CAD build for the part. Positions are in the model's coordinates, mm. Give positions to 0.01 mm unless a question says otherwise; leave off trailing zeros. Loops run counter-clockwise (first coordinate to the right, second up) from the corner with the lowest first, then second, coordinate; pieces in that order, holes last. Notation, with made-up numbers: (39, 2.5) -> (75, 2.5) arc R20 ccw to (75, 34.5) -> close; hole circle Ø7 at (17, -20.75). An arc over 180 degrees is marked (long way). Use one line per item in the form item = value.
Autodesk Inventor part; units mm, degrees
ref_plane "YZ Plane" through (0, 0, 0) normal (1, 0, 0) x (0, 1, 0)
ref_plane "XZ Plane" through (0, 0, 0) normal (0, 1, 0) x (-1, 0, 0)
ref_plane "XY Plane" through (0, 0, 0) normal (0, 0, 1) x (1, 0, 0)
sketch "Sketch1" plane through (0, 0, 0) normal (0, 0, 1) x (1, 0, 0)
  line L0 (-8.5, 20) -> (8.5, 20)
  line L1 (8.5, 20) -> (8.5, -20)
  line L2 (8.5, -20) -> (-8.5, -20)
  line L3 (-8.5, -20) -> (-8.5, 20)
  point P0 (0, 0)
  point P1 (-8.5, 0)
  point P2 (0, 20)
  dimension "d0" = 40
  dimension "d1" = 17
extrude "Extrusion1" add sketch "Sketch1" along normal blind 15
sketch "Sketch2" plane through (-8.5, -20, 0) normal (-1, 0, 0) x (0, 0, 1)
  circle A0 centre (0, 20) radius 5.15
  line L0 (0, 40) -> (0, 0)
  dimension "d5" = 10.3
  dimension "d8" = 0
extrude "Extrusion2" cut sketch "Sketch2" against normal through all
sketch "Sketch3" plane through (0, 0, 0) normal (0, 0, -1) x (-1, 0, 0)
  line L0 (-8.5, 5.15) -> (-8.5, 20)
  line L1 (-8.5, -20) -> (-8.5, -5.15)
  line L2 (8.5, -20) -> (-8.5, -20)
  line L3 (-8.5, 20) -> (8.5, 20)
  point P0 (0, 0)
  point P1 (0, -12.575)
  point P2 (0, 12.575)
  point P3 (-8.5, 12.575)
  point P4 (-8.5, -12.575)
  point P5 (0, -20)
  point P6 (0, 20)
hole "Hole1" at (0, -12.575, 0) at (0, 12.575, 0) direction (0, 0, 1) diameter 5.5 end through all
fillet "Fillet1" radius 2 2 edges at (0, -20, 15) (0, 20, 15)
properties part number "0008-10-010 Fixare AxaX"
1. Cut at A-A, the plane z = 2. Write the cut outline in (x, y) (3 decimals).
Result sheet:
outline = (-8.5, -20) -> (8.5, -20) -> (8.5, -4.746) -> (-8.5, -4.746) -> close; (-8.5, 4.746) -> (8.5, 4.746) -> (8.5, 20) -> (-8.5, 20) -> close; hole circle Ø5.5 at (0, -12.575); hole circle Ø5.5 at (0, 12.575)
2. Cut at D-D, the plane z = 6.5. Write the cut outline in (x, y) (3 decimals), then the cut area to 3 significant figures.
Result sheet:
outline = (-8.5, -20) -> (8.5, -20) -> (8.5, 20) -> (-8.5, 20) -> close; hole circle Ø5.5 at (0, -12.575); hole circle Ø5.5 at (0, 12.575)
area = 632 mm^2
3. Mould opens along Y. For faces 1 (the flat face through (0, 16, 0)), 2 (the cylindrical face through (1.67, 10.39, 7.6)), 3 (the flat face through (0, 20, 6)), 4 (the cylindrical face through (-0.12, -19.43, 14.4)) say: pulls with the +Y half, pulls with the -Y half, needs draft (parallel to the pull), parting line crosses it, or undercut.
Result sheet:
face_1 = needs draft
face_2 = undercut
face_3 = pulls with the +Y half
face_4 = pulls with the -Y half
4. Drop flat-ended pins along their axis: P1, Ø4, axis at x = -6.5, y = -9, coming from the -Z side; P2, Ø3.5, axis at x = 0, y = -12.575, coming from the -Z side. Give the stop position or say it passes through.
Result sheet:
P1 = 0
P2 = through
5. Drill centre lines: line 1 (Y direction, x = 0, z = 9.25) (3 decimals); line 2 (Y direction, x = -2.5, z = 14); line 3 (X direction, y = -12, z = 3.75). Where is each one in solid material? Low to high.
Result sheet:
line_1 = -20 to -15.325, -9.825 to 9.825, 15.325 to 20
line_2 = -19.73 to -13.72, -11.43 to 11.43, 13.72 to 19.73
line_3 = -8.5 to -2.69, 2.69 to 8.5
6. Cut at B-B, the plane x = 0. Write the cut outline in (y, z) (3 decimals).
Result sheet:
outline = (-20, 0) -> (-15.325, 0) -> (-15.325, 15) -> (-18, 15) arc R2 ccw to (-20, 13) -> close; (-9.825, 0) -> (-5.15, 0) arc R5.15 cw to (5.15, 0) -> (9.825, 0) -> (9.825, 15) -> (-9.825, 15) -> close; (15.325, 0) -> (20, 0) -> (20, 13) arc R2 ccw to (18, 15) -> (15.325, 15) -> close
7. Cut at C-C, the plane x = 4.25. Write the cut outline in (y, z), then the cut area to 3 significant figures.
Result sheet:
outline = (-20, 0) -> (-5.15, 0) arc R5.15 cw to (5.15, 0) -> (20, 0) -> (20, 13) arc R2 ccw to (18, 15) -> (-18, 15) arc R2 ccw to (-20, 13) -> close
area = 557 mm^2
